Could you check a few things on this model? Use its own coordinates, in mm. Give positions to 0.01 mm unless a question says otherwise; leave off trailing zeros. Loops run counter-clockwise (first coordinate to the right, second up) from the corner with the lowest first, then second, coordinate; pieces in that order, holes last. Notation, with made-up numbers: (45, 52) - (80, 52) arc R14 ccw to (80, 69) - close; hole circle Ø7 at (-6, 86.5). An arc over 180 degrees is marked (long way). Write each question's results on one line, items separated by ' | '. Start each with the question number.
(1) I need wall thicknesses on line 1 (Y direction, x = -97.85, z = 1.35); line 2 (Y direction, x = -151, z = 3.75); line 3 (Y direction, x = 151, z = 2.75). Which ranges of each line are inside material? Lowest first, please.
(2) Suppose I cut it at C-C (z = 2.25). Count the separate pieces of the cut face and the enclosed holes in it, and give its area (3 significant figures).
(3) Suppose I cut it at A-A (y = 50). Please give me the cut outline in (x, z), and give its area (3 significant figures).
(4) Suppose I cut it at B-B (x = -84.5). Please give me the cut outline in (y, z), and give its area (3 significant figures).
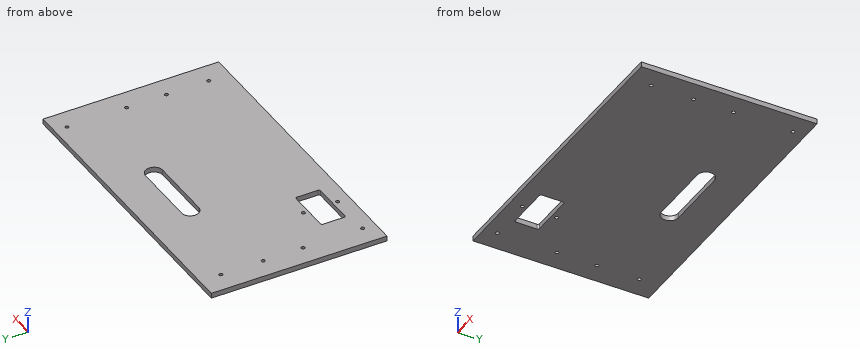
from build123d import *

# Parameters (mm, degrees)
ESBO_O1_W                    = 350
ESBO_O1_H                    = 205
RESSALTO_EXTRUS_O1_DEPTH     = 6
CORTE_EXTRUS_O1_DEPTH        = 203.897141429
ESBO_O3_R                    = 2.1
CORTE_EXTRUS_O2_DEPTH        = 203.897141429
FURO_DE_DI_METRO_4_2_4_2_1_D = 4.2


with BuildPart() as part:
    # Esboço1 → Ressalto-extrusão1 (new body)
    with BuildSketch(Plane.XY):
        Rectangle(ESBO_O1_W, ESBO_O1_H)
    extrude(amount=RESSALTO_EXTRUS_O1_DEPTH)

    # Esboço2 → Corte-extrusão1 (cut, through all)
    with BuildSketch(Plane.XY.offset(6)):
        with BuildLine():
            Line((-37.5, 60), (37.5, 60))
            ThreePointArc((37.5, 60), (47.5, 50), (37.5, 40))
            Line((37.5, 40), (-37.5, 40))
            ThreePointArc((-37.5, 40), (-47.5, 50), (-37.5, 60))
        make_face()
    extrude(amount=-CORTE_EXTRUS_O1_DEPTH, mode=Mode.SUBTRACT)

    # Esboço3 → Corte-extrusão2 (cut, through all)
    with BuildSketch(Plane.XY.offset(6)):
        with Locations((-97.85, -48.25)):
            Circle(ESBO_O3_R)
        with Locations((-97.85, -88.25)):
            Circle(ESBO_O3_R)
        with BuildLine():
            Line((-123, -82.5), (-72.7, -82.5))
            ThreePointArc((-72.7, -82.5), (-71.285786438, -81.914213562), (-70.7, -80.5))
            Line((-70.7, -80.5), (-70.7, -56))
            ThreePointArc((-70.7, -56), (-71.285786438, -54.585786438), (-72.7, -54))
            Line((-72.7, -54), (-123, -54))
            ThreePointArc((-123, -54), (-124.414213562, -54.585786438), (-125, -56))
            Line((-125, -56), (-125, -80.5))
            ThreePointArc((-125, -80.5), (-124.414213562, -81.914213562), (-123, -82.5))
        make_face()
    extrude(amount=-CORTE_EXTRUS_O2_DEPTH, mode=Mode.SUBTRACT)

    # Furo de diâmetro Ø4.2 (4.2)1 (through all)
    with Locations(Plane.XY.offset(6)):
        with Locations((-151, -87.5), (-151, -18), (151, -28), (151, -77.5), (151, 88), (151, 18.5), (-151, 78), (-151, 28.5)):
            Hole(FURO_DE_DI_METRO_4_2_4_2_1_D / 2)


solid = part.part
Output values:
1) line 1: -102.5 to -90.35, -86.15 to -82.5, -54 to -50.35, -46.15 to 102.5 | line 2: -102.5 to -89.6, -85.4 to -20.1, -15.9 to 26.4, 30.6 to 75.9, 80.1 to 102.5 | line 3: -102.5 to -79.6, -75.4 to -30.1, -25.9 to 16.4, 20.6 to 85.9, 90.1 to 102.5
2) separate pieces: 1 | enclosed holes: 12 | area: 68,300 mm2
3) outline: (-175, 0) - (-47.5, 0) - (-47.5, 6) - (-175, 6) - close; (47.5, 0) - (175, 0) - (175, 6) - (47.5, 6) - close | area: 1,530 mm2
4) outline: (-102.5, 0) - (-82.5, 0) - (-82.5, 6) - (-102.5, 6) - close; (-54, 0) - (102.5, 0) - (102.5, 6) - (-54, 6) - close | area: 1,060 mm2
